For this review, take the finished solid that the model builds, in its own axes (mm). Face numbers are marked on the shaded views. Round coordinates to 2 decimals unless told otherwise and drop trailing zeros. One line per question, with ' | ' between items.
Solid Edge part; units mm, degrees
sketch "Sketch1" plane through (0, 0, 0) normal (0, 0, 1) x (1, 0, 0)
  line L0 (-12.225, -10) -> (12.225, -10)
  arc A0 (-22.225, 0) -> (22.225, 0) centre (0, 0) cw
  arc A1 (22.225, 0) -> (12.225, -10) centre (12.225, 0) cw
  arc A2 (-12.225, -10) -> (-22.225, 0) centre (-12.225, 0) cw
extrude "Protrusion1" add sketch "Sketch1" along normal blind 4
sketch "Sketch2" plane through (0, 0, 0) normal (0, 0, 1) x (1, 0, 0)
  line L0 (2.05, -3.6407) -> (17.6546, -2.3823)
  arc A0 (17.6546, -2.3823) -> (17.6546, 2.3823) centre (17.4625, 0) ccw
  line L1 (17.6546, 2.3823) -> (2.05, 3.6407)
  line L2 (2.05, 3.6407) -> (2.05, 6.35)
  arc A1 (2.05, 6.35) -> (-2.05, 6.35) centre (0, 6.35) ccw
  line L3 (-2.05, 6.35) -> (-2.05, 3.6407)
  line L4 (-2.05, 3.6407) -> (-17.6546, 2.3823)
  arc A2 (-17.6546, 2.3823) -> (-17.6546, -2.3823) centre (-17.4625, 0) ccw
  line L5 (-17.6546, -2.3823) -> (-2.05, -3.6407)
  line L6 (-2.05, -3.6407) -> (-2.05, -6.35)
  arc A3 (-2.05, -6.35) -> (2.05, -6.35) centre (0, -6.35) ccw
  line L7 (2.05, -6.35) -> (2.05, -3.6407)
extrude "ExtrudedCutout_1" cut sketch "Sketch2" along normal blind 2
sketch "Sketch3" plane through (0, 6.1125, 0) normal (0, 0, -1) x (1, 0, 0)
  line L0 (-13, 12.7485) -> (-9, 12.7485)
  line L1 (-9, 12.7485) -> (-9, 10.7485)
  line L2 (-9, 10.7485) -> (-13, 10.7485)
  line L3 (-13, 10.7485) -> (-13, 12.7485)
  line L4 (-13, -0.5235) -> (-13, 1.4765)
  line L5 (-13, 1.4765) -> (-9, 1.4765)
  line L6 (-9, 1.4765) -> (-9, -0.5235)
  line L7 (-9, -0.5235) -> (-13, -0.5235)
  line L8 (13, -0.5235) -> (9, -0.5235)
  line L9 (9, -0.5235) -> (9, 1.4765)
  line L10 (9, 1.4765) -> (13, 1.4765)
  line L11 (13, 1.4765) -> (13, -0.5235)
  line L12 (9, 12.7485) -> (13, 12.7485)
  line L13 (13, 12.7485) -> (13, 10.7485)
  line L14 (13, 10.7485) -> (9, 10.7485)
  line L15 (9, 10.7485) -> (9, 12.7485)
extrude "Cutout1" cut sketch "Sketch3" against normal through all
fillet "Round_1" radius 1 8 edges at (11, 4.636, 0) (11, -4.636, 0) (11, -4.636, 4) (11, 4.636, 4) (-11, 4.636, 4) (-11, -4.636, 4) (-11, -4.636, 0) (-11, 4.636, 0)
sketch "Sketch4" plane through (0, 0, 0) normal (0, -1, 0) x (1, 0, 0)
  line L0 (-22.225, 1) -> (-21.225, 1)
  line L1 (-22.225, 3) -> (-22.225, 1)
  line L2 (-21.225, 3) -> (-22.225, 3)
  arc A0 (-21.225, 3) -> (-21.225, 1) centre (-21.225, 2) cw
revolve "RevolvedCutout_1" cut sketch "Sketch4" angle 180 about axis through (0, 0, 0) along (0, 0, -1)
sketch "Sketch5" plane through (-21.475, 0, 2) normal (0, 1, 0) x (-1, 0, 0)
  circle A0 centre (-0.25, 0) radius 0.75
extrude "Cutout2" cut sketch "Sketch5" against normal through all
mirror "Mirror1" about plane through (0, 0, 0) normal (1, 0, 0) of "Cutout2"
sketch "Sketch6" plane through (0, 0, 0) normal (0, 0, -1) x (-1, 0, 0)
  circle A0 centre (0, 0) radius 3.9688
extrude "Cutout4" cut sketch "Sketch6" against normal up to vertex (4 mm away)
sketch "Sketch7" plane through (0, 6.1125, 0) normal (0, 0, -1) x (1, 0, 0)
  line L0 (-9, 10.7485) -> (-9, 1.4765)
  line L1 (-9, 1.4765) -> (-13, 1.4765)
  line L2 (-13, 1.4765) -> (-13, 10.7485)
  line L3 (-13, 10.7485) -> (-9, 10.7485)
  line L4 (9, 10.7485) -> (9, 1.4765)
  line L5 (9, 1.4765) -> (13, 1.4765)
  line L6 (13, 1.4765) -> (13, 10.7485)
  line L7 (13, 10.7485) -> (9, 10.7485)
extrude "Cutout5" cut sketch "Sketch7" against normal up to vertex (2 mm away)
sketch "Sketch8" plane through (0, 6.1125, 4) normal (0, 0, 1) x (1, 0, 0)
  circle A0 centre (15.5, -13.6125) radius 0.75
  circle A1 centre (3, -13.6125) radius 0.75
extrude "ExtrudedCutout_9" cut sketch "Sketch8" against normal blind 4
mirror "Mirror2" about plane through (0, 0, 0) normal (1, 0, 0) of "ExtrudedCutout_9"
sketch "Sketch9" plane through (0, 6.1125, 0) normal (0, 0, -1) x (1, 0, 0)
  line L0 (16.1495, 13.2375) -> (17.1495, 14.9696)
  line L1 (15.8505, 15.7196) -> (17.1495, 14.9696)
  line L2 (14.8505, 13.9875) -> (15.8505, 15.7196)
  line L3 (16.1495, 13.2375) -> (14.8505, 13.9875)
extrude "ExtrudedCutout_12" cut sketch "Sketch9" against normal blind 1
mirror "Mirror3" about plane through (0, 0, 0) normal (1, 0, 0) of "ExtrudedCutout_12"
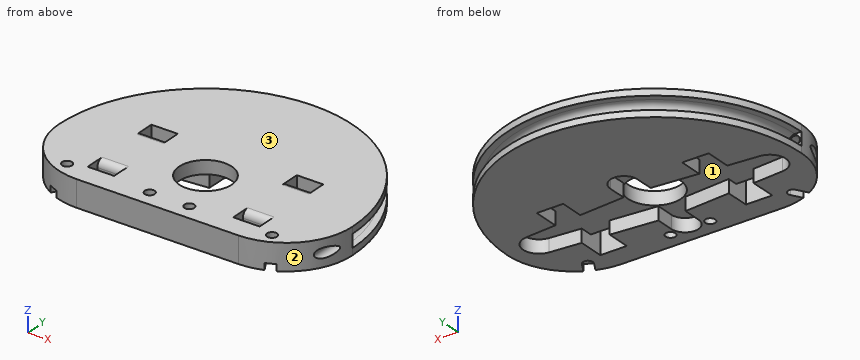
(1) We need section A-A on x = 3. Give the number of separate pieces and of enclosed holes in the cut face, plus the area to 3 significant figures.
Output values:
separate pieces: 3 | enclosed holes: 0 | area: 93.8 mm^2
(2) Insertion check: pin 1 (0.9 mm diameter, centred on x = 3, y = -7.5, fed in from -Z) (3 decimals); pin 2 (2 mm diameter, centred on x = -10.5, y = 0.5, fed in from -Z); pin 3 (8 mm diameter, centred on x = 3, y = -2, fed in from +Z); pin 4 (2 mm diameter, centred on x = 16, z = 2.5, fed in from +Y). Each pin has a flat end and moves straight along its axis. Give the tip position at first contact, or say it passes through.
Output values:
pin 1: through | pin 2: z = 2 | pin 3: z = 4 | pin 4: y = 16.28
(3) Mouldability with a two-part tool opening along Y and no side actions: class the marked faces 1, 2 and 3 as released by +Y, released by -Y, zero draft, split by the parting line, or undercut.
Output values:
face 1: undercut | face 2: released by -Y | face 3: zero draft
(4) For probe 1 along Y at (x, z) = (3, 3.05); probe 2 along X at (y, z) = (6, 3.2); probe 3 along Y at (x, z) = (15.5, 1.9), list the stretches that pass through material, from the lowest coordinate up. Write a range as [from, to].
Output values:
probe 1: [-10, -8.25], [-6.75, -2.6], [2.6, 22.02] | probe 2: [-21.4, -13], [-9, 9], [13, 21.4] | probe 3: [-9.45, -8.25], [-6.75, -2.56], [2.56, 13]
